Can you work these out from the model? Positions are in its coordinate system, mm. A direction names the side the tool comes from. Coordinates: 2 decimals unless noted, no trailing zeros. Order: outer loops, then holes, each group sorted by start corner. A loop starts at its lowest first (then second) coordinate and runs counter-clockwise, first axis right, second up. Notation, with made-up numbers: (25.5, 70.25) - (63.5, 70.25) arc R27 cw to (63.5, 100.25) - close; hole circle Ø1 at (11.5, -19). An arc over 180 degrees is marked (long way). Return JSON: item names as keys, results as strings. Group by question number.
1) For pin 1 Ø4.5 at (y, z) = (-16.27, 8) entering from -X; pin 2 Ø3 at (x, y) = (40, 25) entering from +Z, each with a flat end and sliding along its axis, tell me the tip position at first contact or that it passes through.
2) Imagine slicing it at A-A (z = 4.5). Write out the boundary of the cut face in (x, y), and give its area (3 significant figures).
3) Which directions (+Z, -Z, +X, -X, +Y, -Y) give clear straight access to the entire face, cutting with the end or side of a thin tool? Please do faces 5 (the face through (44.19, -31.2, 7.93)), 6 (the face through (51.583, -14.288, 6.479)).
4) Imagine slicing it at D-D (x = -2). Write out the boundary of the cut face in (y, z), and give its area (3 significant figures).
5) Imagine slicing it at B-B (x = 20.5). Write out the boundary of the cut face in (y, z).
6) Imagine slicing it at C-C (y = -15.5). Write out the boundary of the cut face in (x, z), and give its area (3 significant figures).
7) If I drill on line 1 along X through (y, z) = (17, 4.75); line 2 along X through (y, z) = (31.75, 8); line 3 along X through (y, z) = (-19, 4.5), over which ranges is the centre line in solid material (lowest first)?
8) If we mould it in two halves opening along Y, with no side actions, what happens to faces 1 (the face through (-8, 13.728, 8)), 2 (the face through (17, -41.272, 6)), 3 (the face through (19, 28.728, 8)), 4 (the face through (23, 33.728, 6))? For each: pulls with the +Y half, pulls with the -Y half, needs draft (parallel to the pull), parting line crosses it, or undercut.
```python
from build123d import *

# Parameters (mm, degrees)
BOSS_EXTRU_1_DEPTH        = 13
COQUE1_T                  = -5
COQUE1_THICKNESS_2_FACE_W = 65
COQUE1_THICKNESS_2_FACE_H = 65
COQUE1_THICKNESS_2_DEPTH  = 2
ENL_V_MAT_EXTRU_1_REACH   = 88.587
ESQUISSE2_R               = 2.5
ENL_V_MAT_EXTRU_2_REACH   = 95.396
ESQUISSE3_R               = 2.5
ESQUISSE4_W               = 15
ESQUISSE4_H               = 15
BOSS_EXTRU_2_DEPTH        = 10
ESQUISSE5_R               = 11.5
ENL_V_MAT_EXTRU_3_DEPTH   = 13


with BuildPart() as part:
    # Esquisse1 → Boss.-Extru.1 (new body)
    with BuildSketch(Plane.XY):
        Polygon((44.118436308, 33.728448276), (54.118436308, 33.728448276), (54.118436308, 23.728448276), (54.118436308, -41.271551724), (-20.881563692, -41.271551724), (-20.881563692, 33.728448276), align=None)
    extrude(amount=BOSS_EXTRU_1_DEPTH)

    # Coque1
    coque1_openings = [part.faces().sort_by_distance(p)[0] for p in [
        (16.618436308, -3.771551724, 13),
    ]]
    offset(amount=COQUE1_T, openings=coque1_openings, kind=Kind.INTERSECTION)

    # Coque1 thickness 2 face (on inner face of the shell) → Coque1 thickness 2 (cut)
    with BuildSketch(Plane(origin=(16.618436308, -3.771551724, 5), x_dir=(-1, 0, 0), z_dir=(0, 0, -1))):
        Rectangle(COQUE1_THICKNESS_2_FACE_W, COQUE1_THICKNESS_2_FACE_H)
    extrude(amount=COQUE1_THICKNESS_2_DEPTH, mode=Mode.SUBTRACT)

    # Enlèv. mat.-Extru.1: up to this face of the body (flat: up to its plane)
    enl_v_mat_extru_1_end = Plane(part.part.faces().sort_by_distance((54.118436308, -3.771551724, 6.5))[0])
    # Esquisse2 → Enlèv. mat.-Extru.1 (cut, up to the picked face)
    with BuildSketch(Plane.ZY.offset(20.881563692), mode=Mode.PRIVATE) as enl_v_mat_extru_1_sk1:
        with Locations(Location((8, -16.271551724, 0), (0, 0, 270))):
            Circle(ESQUISSE2_R)
    enl_v_mat_extru_1_tool1 = split(extrude(enl_v_mat_extru_1_sk1.sketch, amount=-ENL_V_MAT_EXTRU_1_REACH, mode=Mode.PRIVATE), bisect_by=enl_v_mat_extru_1_end, keep=Keep.BOTH, mode=Mode.PRIVATE)
    # Esquisse2 → Enlèv. mat.-Extru.1 (cut, up to the picked face)
    with BuildSketch(Plane.ZY.offset(20.881563692), mode=Mode.PRIVATE) as enl_v_mat_extru_1_sk2:
        with Locations(Location((8, 8.728448276, 0), (0, 0, 270))):
            Circle(ESQUISSE2_R)
    enl_v_mat_extru_1_tool2 = split(extrude(enl_v_mat_extru_1_sk2.sketch, amount=-ENL_V_MAT_EXTRU_1_REACH, mode=Mode.PRIVATE), bisect_by=enl_v_mat_extru_1_end, keep=Keep.BOTH, mode=Mode.PRIVATE)
    add(enl_v_mat_extru_1_tool1.solids().sort_by(Axis((-20.881564, -16.271552, 8), (1, 0, 0)))[0], mode=Mode.SUBTRACT)
    add(enl_v_mat_extru_1_tool2.solids().sort_by(Axis((-20.881564, 8.728448, 8), (1, 0, 0)))[0], mode=Mode.SUBTRACT)

    # Enlèv. mat.-Extru.2: up to this face of the body (flat: up to its plane)
    enl_v_mat_extru_2_end = Plane(part.part.faces().sort_by_distance((16.618436308, 33.728448276, 6.5))[0])
    # Esquisse3 → Enlèv. mat.-Extru.2 (cut, up to the picked face)
    with BuildSketch(Plane.XZ.offset(41.271551724), mode=Mode.PRIVATE) as enl_v_mat_extru_2_sk1:
        with Locations(Location((4.118436308, 8, 0), (0, 0, 270))):
            Circle(ESQUISSE3_R)
    enl_v_mat_extru_2_tool1 = split(extrude(enl_v_mat_extru_2_sk1.sketch, amount=-ENL_V_MAT_EXTRU_2_REACH, mode=Mode.PRIVATE), bisect_by=enl_v_mat_extru_2_end, keep=Keep.BOTH, mode=Mode.PRIVATE)
    # Esquisse3 → Enlèv. mat.-Extru.2 (cut, up to the picked face)
    with BuildSketch(Plane.XZ.offset(41.271551724), mode=Mode.PRIVATE) as enl_v_mat_extru_2_sk2:
        with Locations(Location((29.118436308, 8, 0), (0, 0, 270))):
            Circle(ESQUISSE3_R)
    enl_v_mat_extru_2_tool2 = split(extrude(enl_v_mat_extru_2_sk2.sketch, amount=-ENL_V_MAT_EXTRU_2_REACH, mode=Mode.PRIVATE), bisect_by=enl_v_mat_extru_2_end, keep=Keep.BOTH, mode=Mode.PRIVATE)
    add(enl_v_mat_extru_2_tool1.solids().sort_by(Axis((4.118436, -41.271552, 8), (0, 1, 0)))[0], mode=Mode.SUBTRACT)
    add(enl_v_mat_extru_2_tool2.solids().sort_by(Axis((29.118436, -41.271552, 8), (0, 1, 0)))[0], mode=Mode.SUBTRACT)

    # Esquisse4 → Boss.-Extru.2 (add)
    with BuildSketch(Plane.XY.offset(3)):
        Polygon((-15.881563692, -26.271551724), (-5.881563692, -36.271551724), (-15.881563692, -36.271551724), align=None)
        Polygon((49.118436308, 28.728448276), (49.118436308, 18.728448276), (39.118436308, 28.728448276), align=None)
        Polygon((49.118436308, -36.271551724), (49.118436308, -26.271551724), (39.118436308, -36.271551724), align=None)
        with Locations((-8.381563692, 21.228448276)):
            Rectangle(ESQUISSE4_W, ESQUISSE4_H)
    extrude(amount=BOSS_EXTRU_2_DEPTH)

    # Esquisse5 → Enlèv. mat.-Extru.3 (cut)
    with BuildSketch(Plane.XY.offset(13)):
        with Locations((-20.881563692, 33.728448276)):
            Circle(ESQUISSE5_R)
    extrude(amount=-ENL_V_MAT_EXTRU_3_DEPTH, mode=Mode.SUBTRACT)


solid = part.part
```
Calculated:
{
 "1": {"pin 1": "through", "pin 2": "z = 3"},
 "2": {"outline": "(-20.88, -41.27) - (54.12, -41.27) - (54.12, 33.73) - (-9.38, 33.73) arc R11.5 cw to (-20.88, 22.23) - close; hole (-15.88, -26.27) - (-5.88, -36.27) - (39.12, -36.27) - (49.12, -26.27) - (49.12, 18.73) - (39.12, 28.73) - (-0.88, 28.73) - (-0.88, 13.73) - (-15.88, 13.73) - close", "area": "1,670 mm2"},
 "3": {"face 5": "+Z", "face 6": "+X, -X"},
 "4": {"outline": "(-41.27, 0) - (33.73, 0) - (33.73, 13) - (13.73, 13) - (13.73, 3) - (-36.27, 3) - (-36.27, 13) - (-41.27, 13) - close", "area": "475 mm2"},
 "5": {"outline": "(-41.27, 0) - (33.73, 0) - (33.73, 13) - (28.73, 13) - (28.73, 3) - (-36.27, 3) - (-36.27, 13) - (-41.27, 13) - close"},
 "6": {"outline": "(-20.88, 0) - (54.12, 0) - (54.12, 5.62) - (49.12, 5.62) - (49.12, 3) - (-15.88, 3) - (-15.88, 5.62) - (-20.88, 5.62) - close; (-20.88, 10.38) - (-15.88, 10.38) - (-15.88, 13) - (-20.88, 13) - close; (49.12, 10.38) - (54.12, 10.38) - (54.12, 13) - (49.12, 13) - close", "area": "277 mm2"},
 "7": {"line 1": "-20.88 to -0.88, 49.12 to 54.12", "line 2": "-9.55 to 1.62, 6.62 to 26.62, 31.62 to 54.12", "line 3": "-20.88 to -15.88, 49.12 to 54.12"},
 "8": {"face 1": "undercut", "face 2": "pulls with the -Y half", "face 3": "undercut", "face 4": "pulls with the +Y half"}
}
